Geometry check sheet. Reference: the model listing, model coordinates, mm. A direction names the side the tool comes from. Coordinates: 2 decimals unless noted, no trailing zeros. Loops run counter-clockwise (first coordinate to the right, second up) from the corner with the lowest first, then second, coordinate; pieces in that order, holes last. Notation, with made-up numbers: (72.25, -34.75) - (79.25, -34.75) arc R26 ccw to (79.25, -5.75) - close; hole circle Ø1 at (-19, 41.25). An arc over 180 degrees is marked (long way). One line per item, written item: value.
Autodesk Fusion 360 part; units mm, degrees
sketch "Sketch1" plane through (0, 0, 0) normal (0, 1, 0) x (1, 0, 0)
  line L0 (5, 0) -> (-542, 0)
  line L1 (5, 540) -> (-561, 540)
  line L2 (5, 540) -> (5, 295)
  line L3 (5, 540) -> (5, 295)
  line L4 (5, 295) -> (-33.6787, 295)
  line L5 (5, 235) -> (-33.6787, 235)
  line L6 (-557, 59.3636) -> (-542, 0)
  arc A0 (-33.6787, 295) -> (-33.6787, 235) centre (-33.6787, 265) ccw
  line L7 (5, 0) -> (5, 235)
  line L8 (5, 295) -> (5, 540)
  line L9 (-561, 540) -> (-557, 59.3636)
  dimension "d1" = 540
  dimension "d2" = 547
  dimension "d3" = 566
  dimension "d4" = 245
  dimension "d5" = 305
  dimension "d11" = 60
  dimension "d12" = 562
extrude "Extrude1" add sketch "Sketch1" along normal blind 12.5
equation "d3 = 562 mm + 4 mm"
(1) Release check for a two-part mould opening along Z. For faces 1 (the face through (-282, 12.5, -274)), 2 (the face through (-265, 6, 0)), 3 (the face through (-14, 6, -235)) record: pulls with the +Z half, pulls with the -Z half, needs draft (parallel to the pull), parting line crosses it, or undercut.
Reply:
face 1: needs draft
face 2: pulls with the +Z half
face 3: undercut
(2) Cross-section at A-A on x = -51.5. Record the cut outline in (y, z).
Reply:
outline: (0, -540) - (12.5, -540) - (12.5, -289.13) - (0, -289.13) - close; (0, -240.87) - (12.5, -240.87) - (12.5, 0) - (0, 0) - close
(3) Material ranges on probe 1 along X at (y, z) = (4.75, -60.5); probe 2 along X at (y, z) = (7, -84.5), recorded low to high. Write a range as from..to.
Reply:
probe 1: -557.01..5
probe 2: -557.21..5
(4) Access from +Z, -Z, +X, -X, +Y, -Y to the whole of each face (thin tool, end or side, straight path). Record for faces 4 (the face through (-14, 6, -295)), 5 (the face through (5, 6, -419)).
Reply:
face 4: +X, +Y, -Y
face 5: +Z, -Z, +X, +Y, -Y
(5) Go/stop test with flat-tipped pins: pin 1 Ø1.5 at (x, y) = (-481, 1.5) entering from +Z; pin 2 Ø4 at (y, z) = (4.5, -277) entering from +X. Record where each tip stops, or that it passes through.
Reply:
pin 1: z = 0
pin 2: x = -60.21
(6) Cross-section at B-B on y = 6. Record the cut outline in (x, z), and give its area (3 significant figures).
Reply:
outline: (-561, -540) - (5, -540) - (5, -295) - (-33.68, -295) arc R30 cw to (-33.68, -235) - (5, -235) - (5, 0) - (-542, 0) - (-557, -59.36) - close
area: 300,000 mm2
(7) Cross-section at C-C on z = -265. Record the cut outline in (x, y).
Reply:
outline: (-558.71, 0) - (-63.68, 0) - (-63.68, 12.5) - (-558.71, 12.5) - close
